```python
from build123d import *

# Parameters (mm, degrees)
F0_W     = 100
F0_H     = 60
F1_DEPTH = 50
F2_T     = -2.5
F3_R     = 1.75
F3_R_2   = 0.75
F4_DEPTH = 10
F5_R     = 5


with BuildPart() as f1:
    # F0 (on Front) → F1 (new body)
    with BuildSketch(Plane.XZ):
        with Locations((-64.083846, 18.250474)):
            Rectangle(F0_W, F0_H)
    extrude(amount=F1_DEPTH)

    # F2
    f2_openings = [f1.faces().sort_by_distance(p)[0] for p in [
        (-64.083846, -50, 18.250474),
    ]]
    offset(amount=F2_T, openings=f2_openings)

    # F3 (on face) → F4 (join)
    with BuildSketch(Plane.XZ.offset(2.5)):
        with Locations((-96.083846, 38.250474)):
            Circle(F3_R)
        with Locations((-96.083846, 38.250474)):
            Circle(F3_R_2, mode=Mode.SUBTRACT)
        with Locations((-31.583846, 38.250474)):
            Circle(F3_R)
        with Locations((-31.583846, 38.250474)):
            Circle(F3_R_2, mode=Mode.SUBTRACT)
        with Locations((-96.583846, -2.249526)):
            Circle(F3_R)
        with Locations((-96.583846, -2.249526)):
            Circle(F3_R_2, mode=Mode.SUBTRACT)
        with Locations((-31.583846, -1.749526)):
            Circle(F3_R)
        with Locations((-31.583846, -1.749526)):
            Circle(F3_R_2, mode=Mode.SUBTRACT)
    extrude(amount=F4_DEPTH)

    # F5
    f5_edges = [f1.edges().sort_by_distance(p)[0] for p in [
        (-114.083846, -25, 48.250474),
        (-114.083846, -25, -11.749526),
        (-14.083846, -25, -11.749526),
        (-14.083846, -25, 48.250474),
    ]]
    fillet(f5_edges, radius=F5_R)


solid = f1.part
```
Check sheet for the modelled part. Datum: model origin and axes. Units: mm. A direction names the side the tool comes from. Round coordinates to 2 decimals unless told otherwise and drop trailing zeros. Loops run counter-clockwise (first coordinate to the right, second up) from the corner with the lowest first, then second, coordinate; pieces in that order, holes last. Notation, with made-up numbers: (70, 79.25) -> (103, 79.25) arc R37 ccw to (103, 116.25) -> close; hole circle Ø5 at (-21.75, -6). An arc over 180 degrees is marked (long way). Write item = value, one per line. Start each with the question number.
1) Sectioned sample at D-D, the plane z = 31.5. Record the cut outline in (x, y), plus the area to 4 significant figures.
2) Thickness scan on probe 1 along Z at (x, y) = (-81.5, -33.5); probe 2 along X at (y, z) = (-15, 3). Record the ranges inside material, lowest first.
3) Sectioned sample at C-C, the plane x = -36. Record the cut outline in (y, z), plus the area to 4 significant figures.
4) Sectioned sample at A-A, the plane y = -9. State how many separate pieces and enclosed holes the cut face has, plus the area to 3 significant figures.
5) Sectioned sample at B-B, the plane y = -29. Record the cut outline in (x, z), plus the area to 3 significant figures.
6) Release check for a two-part mould opening along Z. For faces 1 (the flat face through (-65, -25, 48.25)), 2 (the flat face through (-32, -12.5, 37)), 3 (the cylindrical face through (-15.587, -25.35, -10.324)) record: released by +Z, released by -Z, zero draft, split by the parting line, or undercut.
7) Set-up check for faces 4 (the flat face through (-64, -50, -10)), 5 (the flat face through (-95, -12.5, 38)): record each of +Z, -Z, +X, -X, +Y, -Y from which the full face is reachable in a straight line by a thin tool's end or side.
8) Gauge pin test, flat ends, axial feed: pin 1 Ø10 at (x, z) = (-31.5, 25.5) entering from -Y; pin 2 Ø1.8 at (x, z) = (-31.5, 39) entering from -Y. Record the tip position at first contact, or that the pin passes through.
Results are:
q1.outline = (-114.08, -50) -> (-111.58, -50) -> (-111.58, -2.5) -> (-16.58, -2.5) -> (-16.58, -50) -> (-14.08, -50) -> (-14.08, 0) -> (-114.08, 0) -> close
q1.area = 487.5 mm^2
q2.probe_1 = -11.75 to -9.25, 45.75 to 48.25
q2.probe_2 = -114.08 to -111.58, -16.58 to -14.08
q3.outline = (-50, -11.75) -> (0, -11.75) -> (0, 48.25) -> (-50, 48.25) -> (-50, 45.75) -> (-2.5, 45.75) -> (-2.5, -9.25) -> (-50, -9.25) -> close
q3.area = 387.5 mm^2
q4.separate_pieces = 5
q4.enclosed_holes = 5
q4.area = 785 mm^2
q5.outline = (-114.08, -6.75) arc R5 ccw to (-109.08, -11.75) -> (-19.08, -11.75) arc R5 ccw to (-14.08, -6.75) -> (-14.08, 43.25) arc R5 ccw to (-19.08, 48.25) -> (-109.08, 48.25) arc R5 ccw to (-114.08, 43.25) -> close; hole (-111.58, -9.25) -> (-16.58, -9.25) -> (-16.58, 45.75) -> (-111.58, 45.75) -> close
q5.area = 754 mm^2
q6.face_1 = released by +Z
q6.face_2 = undercut
q6.face_3 = released by -Z
q7.face_4 = +Z, -Z, +X, -X, -Y
q7.face_5 = -Y
q8.pin_1 = -2.5
q8.pin_2 = -12.5
